For this review, take the finished solid that the model builds, in its own axes (mm). Coordinates: 2 decimals unless noted, no trailing zeros. Loops run counter-clockwise (first coordinate to the right, second up) from the corner with the lowest first, then second, coordinate; pieces in that order, holes last. Notation, with made-up numbers: (86, 37.5) -> (123, 37.5) arc R19 cw to (123, 49.5) -> close; hole circle Ø1 at (9.25, -31). An arc over 180 degrees is marked (long way). One line per item, written item: value.
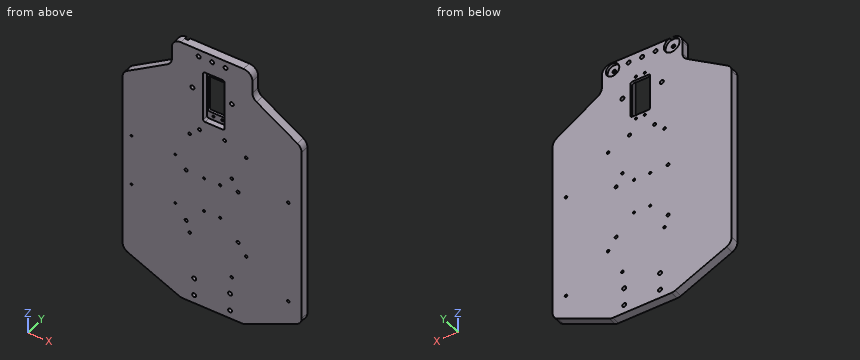
from build123d import *

# Parameters (mm, degrees)
CHASSIS_BASE_SHAPE_DEPTH        = 9.525
M4_CLEARANCE_HOLE1_D            = 4.5
M4_CLEARANCE_HOLE2_D            = 4.5
FILLET1_R                       = 10
SERVO_RECESS_DEPTH              = 6.525
SERVO_CUTOUT_DEPTH              = 4
M3X0_5_SERVO_D                  = 2.5
M2_5_CLEARANCE_ESC_D            = 2.9
M2_5X0_45_TAP_FOR_RPI_D         = 2.05
M2_5X0_45_TAP_FOR_RPI_DEPTH     = 5
M2_5X0_45_TAP_FOR_RPI_TIP       = 0.615882135
SKETCH27_R                      = 8.75
SKETCH27_R_2                    = 7.5
BELLCRANK_POSITIONS_DEPTH       = 3
SKETCH28_R                      = 2
DOWEL_SCREW_CAP_SLOTS_DEPTH     = 2
BATTERY_HOLES_D                 = 3.4
TAP_DRILL_FOR_M3X0_5_TAP1_D     = 2.5
TAP_DRILL_FOR_M3X0_5_TAP1_DEPTH = 9.525


with BuildPart() as part:
    # Sketch2 → Chassis Base Shape (new body)
    with BuildSketch(Plane(origin=(0, 0, 0), x_dir=(1, 0, 0), z_dir=(0, 1, 0))):
        Polygon((-100, -85.226624744), (-45, -120), (-45, -150), (0, -150), (0, 0), (0, 154.8), (-34.83712014, 154.8), (-100, 125.194694643), align=None)
    chassis_base_shape = extrude(amount=CHASSIS_BASE_SHAPE_DEPTH)

    # M4 Clearance Hole1 (through all)
    with Locations(Plane(origin=(0, 0, 0), x_dir=(-1, 0, 0), z_dir=(0, -1, 0))):
        with Locations((15, -142), (0, -142), (22, -102)):
            m4_clearance_hole1 = Hole(M4_CLEARANCE_HOLE1_D / 2)

    # M4 Clearance Hole2 (through all)
    with Locations(Plane(origin=(0, 0, 0), x_dir=(-1, 0, 0), z_dir=(0, -1, 0))):
        with Locations((20, 125.3), (20, 145.3)):
            m4_clearance_hole2 = Hole(M4_CLEARANCE_HOLE2_D / 2)

    # Chassis Base Mirror: Chassis Base Shape, M4 Clearance Hole1, M4 Clearance Hole2 across Right Plane
    add(chassis_base_shape.mirror(Plane(origin=(0, 0, 0), x_dir=(0, 0, -1), z_dir=(1, 0, 0))))
    add(m4_clearance_hole1.mirror(Plane(origin=(0, 0, 0), x_dir=(0, 0, -1), z_dir=(1, 0, 0))), mode=Mode.SUBTRACT)
    add(m4_clearance_hole2.mirror(Plane(origin=(0, 0, 0), x_dir=(0, 0, -1), z_dir=(1, 0, 0))), mode=Mode.SUBTRACT)

    # Fillet1
    fillet1_edges = [part.edges().sort_by_distance(p)[0] for p in [
        (-100, 4.7625, -125.194694643),
        (-34.83712014, 4.7625, -154.8),
        (-45, 4.7625, 150),
        (-45, 4.7625, 120),
        (-100, 4.7625, 85.226624744),
        (100, 4.7625, 85.226624744),
        (100, 4.7625, -125.194694643),
        (34.83712014, 4.7625, -154.8),
        (45, 4.7625, 150),
        (45, 4.7625, 120),
    ]]
    fillet(fillet1_edges, radius=FILLET1_R)

    # Sketch7 → Servo Recess (cut)
    with BuildSketch(Plane(origin=(0, 0, 0), x_dir=(-1, 0, 0), z_dir=(0, -1, 0))):
        with BuildLine():
            Line((-12, -126), (8, -126))
            ThreePointArc((8, -126), (9.414213562, -125.414213562), (10, -124))
            Line((10, -124), (10, -69))
            ThreePointArc((10, -69), (9.414213562, -67.585786438), (8, -67))
            Line((8, -67), (-12, -67))
            ThreePointArc((-12, -67), (-13.414213562, -67.585786438), (-14, -69))
            Line((-14, -69), (-14, -124))
            ThreePointArc((-14, -124), (-13.414213562, -125.414213562), (-12, -126))
        make_face()
    extrude(amount=-SERVO_RECESS_DEPTH, mode=Mode.SUBTRACT)

    # Sketch8 → Servo Cutout (cut, through all)
    with BuildSketch(Plane.XZ.offset(-6.525)):
        with BuildLine():
            Line((-7, 117.5), (11, 117.5))
            ThreePointArc((11, 117.5), (12.414213562, 116.914213562), (13, 115.5))
            Line((13, 115.5), (13, 77.5))
            ThreePointArc((13, 77.5), (12.414213562, 76.085786438), (11, 75.5))
            Line((11, 75.5), (-7, 75.5))
            ThreePointArc((-7, 75.5), (-8.414213562, 76.085786438), (-9, 77.5))
            Line((-9, 77.5), (-9, 115.5))
            ThreePointArc((-9, 115.5), (-8.414213562, 116.914213562), (-7, 117.5))
        make_face()
    extrude(amount=-SERVO_CUTOUT_DEPTH, mode=Mode.SUBTRACT)

    # M3x0.5 Servo (through all)
    with Locations(Plane(origin=(0, 6.525, 0), x_dir=(-1, 0, 0), z_dir=(0, -1, 0))):
        with Locations((3, -71.5), (-7, -71.5), (3, -121.5), (-7, -121.5)):
            Hole(M3X0_5_SERVO_D / 2)

    # M2.5 Clearance ESC (through all)
    with Locations(Plane(origin=(0, 0, 0), x_dir=(-1, 0, 0), z_dir=(0, -1, 0))):
        with Locations((25, 72.8), (-85, -13), (25, -45), (-22, -13), (-22, 104.8), (-38, -45), (-85, 104.8), (-38, 72.8)):
            Hole(M2_5_CLEARANCE_ESC_D / 2)

    # M2.5x0.45 Tap for RPi
    with Locations(Plane(origin=(0, 0, 0), x_dir=(-1, 0, 0), z_dir=(0, -1, 0))):
        with Locations((90, -13.2), (41, -13.2), (41, 44.8), (90, 44.8)):
            Hole(M2_5X0_45_TAP_FOR_RPI_D / 2, depth=M2_5X0_45_TAP_FOR_RPI_DEPTH)
            with Locations((0, 0, -(M2_5X0_45_TAP_FOR_RPI_DEPTH + M2_5X0_45_TAP_FOR_RPI_TIP / 2))):  # 118° drill point
                Cone(0, M2_5X0_45_TAP_FOR_RPI_D / 2, M2_5X0_45_TAP_FOR_RPI_TIP, mode=Mode.SUBTRACT)

    # Sketch27 → Bellcrank Positions (cut)
    with BuildSketch(Plane(origin=(0, 9.525, 0), x_dir=(1, 0, 0), z_dir=(0, 1, 0))):
        with Locations((-33, -141.5)):
            Circle(SKETCH27_R)
        with Locations((33, -141.5)):
            Circle(SKETCH27_R_2)
    extrude(amount=-BELLCRANK_POSITIONS_DEPTH, mode=Mode.SUBTRACT)

    # Sketch28 → Dowel Screw Cap Slots (cut)
    with BuildSketch(Plane(origin=(0, 6.525, 0), x_dir=(1, 0, 0), z_dir=(0, 1, 0))):
        with Locations((-33, -141.5)):
            Circle(SKETCH28_R)
        with Locations((33, -141.5)):
            Circle(SKETCH28_R)
    extrude(amount=-DOWEL_SCREW_CAP_SLOTS_DEPTH, mode=Mode.SUBTRACT)

    # Battery Holes (through all)
    with Locations(Plane(origin=(0, 9.525, 0), x_dir=(1, 0, 0), z_dir=(0, 1, 0))):
        with Locations((-14, -55), (-29, 0), (-29, 60), (29, 60), (29, 0), (14, -55)):
            Hole(BATTERY_HOLES_D / 2)

    # Tap Drill for M3x0.5 Tap1
    with Locations(Plane(origin=(0, 0, 0), x_dir=(-1, 0, 0), z_dir=(0, -1, 0))):
        with Locations((9, 0.8), (-9, 0.8), (9, 39.8), (-9, 39.8)):
            Hole(TAP_DRILL_FOR_M3X0_5_TAP1_D / 2, depth=TAP_DRILL_FOR_M3X0_5_TAP1_DEPTH)


solid = part.part
1. Insertion check: pin 1 Ø3 at (x, z) = (-29, -60) entering from -Y; pin 2 Ø2.5 at (y, z) = (8, 102) entering from +X; pin 3 Ø0.9 at (y, z) = (7.5, 100) entering from -X; pin 4 Ø3 at (x, y) = (-76, 5.5) entering from -Z. Each pin has a flat end and moves straight along its axis. Give the tip position at first contact, or say it passes through.
Return value:
pin 1: passes through
pin 2: stops at x = 75.45
pin 3: stops at x = -77.35
pin 4: stops at z = -136.78
2. Take a section at C-C, the plane x = 75. Give the boundary of the cut face in (y, z) (3 decimals), and give its area (3 significant figures).
Return value:
outline: (0, -136.553) -> (9.525, -136.553) -> (9.525, 101.033) -> (0, 101.033) -> close
area: 2,260 mm2
3. Take a section at A-A, the plane z = 110. Give the boundary of the cut face in (x, y) (3 decimals).
Return value:
outline: (-60.817, 0) -> (-10, 0) -> (-10, 6.525) -> (-9, 6.525) -> (-9, 9.525) -> (-60.817, 9.525) -> close; (13, 6.525) -> (14, 6.525) -> (14, 0) -> (60.817, 0) -> (60.817, 9.525) -> (13, 9.525) -> close
4. Take a section at B-B, the plane x = -64.5. Give the boundary of the cut face in (y, z) (3 decimals).
Return value:
outline: (0, -141.323) -> (9.525, -141.323) -> (9.525, 107.671) -> (0, 107.671) -> close
5. To check wall thickness, follow probe 1 along X at (y, z) = (4.25, -104.8); probe 2 along X at (y, z) = (1.3, -44.8) (3 decimals); probe 3 along Z at (x, y) = (-25, 6). State the ranges of each line that lie inside material, in increasing order. Write a range as from..to.
Return value:
probe 1: x = -100..20.55, 23.45..83.55, 86.45..100
probe 2: x = -100..-91.025, -88.975..-42.025, -39.975..100
probe 3: z = -154.8..-74.25, -71.35..43.55, 46.45..150
